from build123d import *

# Parameters (mm, degrees)
SKETCH2_W                  = 254
SKETCH2_H                  = 88.9
RECTANGLE_EXTRUSION_DEPTH  = 12.7
SKETCH4_W                  = 12.7
SKETCH4_H                  = 12.7
FRONT_FACE_TABS_DEPTH      = 12.7
SKETCH6_R                  = 2.24536
TAB_CURVE_FRONT_BACK_DEPTH = 12.7
SKETCH7_W                  = 12.7
SKETCH7_H                  = 12.7
RIGHT_FACE_TABS_DEPTH      = 12.7
SKETCH8_R                  = 2.24536
TAB_CURVE_LEFT_RIGHT_DEPTH = 12.7
SKETCH9_R                  = 2.5527
NUT_STRIPS_CUT_DEPTH       = 152.471127612


with BuildPart() as part:
    # Sketch2 → Rectangle Extrusion (new body)
    with BuildSketch(Plane(origin=(0, 0, 0), x_dir=(1, 0, 0), z_dir=(0, 1, 0))):
        Rectangle(SKETCH2_W, SKETCH2_H)
    extrude(amount=RECTANGLE_EXTRUSION_DEPTH)

    # Sketch4 → Front Face Tabs (add)
    with BuildSketch(Plane.XY.offset(44.45)):
        with Locations((-63.5, 6.35)):
            Rectangle(SKETCH4_W, SKETCH4_H)
        with Locations((63.5, 6.35)):
            Rectangle(SKETCH4_W, SKETCH4_H)
    front_face_tabs = extrude(amount=FRONT_FACE_TABS_DEPTH)

    # Mirror Rear Face Tabs: Front Face Tabs across plane
    add(front_face_tabs.mirror(Plane.XY))

    # Sketch6 → Tab Curve Front Back (cut)
    with BuildSketch(Plane(origin=(0, 12.7, 0), x_dir=(1, 0, 0), z_dir=(0, 1, 0))):
        with Locations((-71.4375, 46.0375)):
            Circle(SKETCH6_R)
        with Locations((-55.5625, 46.0375)):
            Circle(SKETCH6_R)
        with Locations((55.5625, 46.0375)):
            Circle(SKETCH6_R)
        with Locations((71.4375, 46.0375)):
            Circle(SKETCH6_R)
        with Locations((71.4375, -46.0375)):
            Circle(SKETCH6_R)
        with Locations((55.5625, -46.0375)):
            Circle(SKETCH6_R)
        with Locations((-55.5625, -46.0375)):
            Circle(SKETCH6_R)
        with Locations((-71.4375, -46.0375)):
            Circle(SKETCH6_R)
    extrude(amount=-TAB_CURVE_FRONT_BACK_DEPTH, mode=Mode.SUBTRACT)

    # Sketch7 → Right Face Tabs (add)
    with BuildSketch(Plane(origin=(127, 0, 0), x_dir=(0, 0, -1), z_dir=(1, 0, 0))):
        with Locations((-19.05, 6.35)):
            Rectangle(SKETCH7_W, SKETCH7_H)
        with Locations((19.05, 6.35)):
            Rectangle(SKETCH7_W, SKETCH7_H)
    right_face_tabs = extrude(amount=RIGHT_FACE_TABS_DEPTH)

    # Mirror Left Face Tabs: Right Face Tabs across plane
    add(right_face_tabs.mirror(Plane(origin=(0, 0, 0), x_dir=(0, 0, 1), z_dir=(1, 0, 0))))

    # Sketch8 → Tab Curve Left Right (cut)
    with BuildSketch(Plane(origin=(0, 12.7, 0), x_dir=(1, 0, 0), z_dir=(0, 1, 0))):
        with Locations((128.5875, 26.9875)):
            Circle(SKETCH8_R)
        with Locations((128.5875, 11.1125)):
            Circle(SKETCH8_R)
        with Locations((128.5875, -11.1125)):
            Circle(SKETCH8_R)
        with Locations((128.5875, -26.9875)):
            Circle(SKETCH8_R)
        with Locations((-128.5875, -26.9875)):
            Circle(SKETCH8_R)
        with Locations((-128.5875, -11.1125)):
            Circle(SKETCH8_R)
        with Locations((-128.5875, 11.1125)):
            Circle(SKETCH8_R)
        with Locations((-128.5875, 26.9875)):
            Circle(SKETCH8_R)
    extrude(amount=-TAB_CURVE_LEFT_RIGHT_DEPTH, mode=Mode.SUBTRACT)

    # Sketch9 → Nut Strips Cut (cut, through all)
    with BuildSketch(Plane.XZ):
        with Locations(Location((-107.95, 38.1, 0), (0, 0, 270))):
            Circle(SKETCH9_R)
        with Locations(Location((-120.65, 25.4, 0), (0, 0, 270))):
            Circle(SKETCH9_R)
        with Locations(Location((-120.65, 6.35, 0), (0, 0, 270))):
            Circle(SKETCH9_R)
        with Locations(Location((-120.65, -12.7, 0), (0, 0, 270))):
            Circle(SKETCH9_R)
        with Locations(Location((-120.65, -31.75, 0), (0, 0, 270))):
            Circle(SKETCH9_R)
        with Locations(Location((-88.9, 38.1, 0), (0, 0, 270))):
            Circle(SKETCH9_R)
        with Locations(Location((-69.85, 38.1, 0), (0, 0, 270))):
            Circle(SKETCH9_R)
        with Locations(Location((-50.8, 38.1, 0), (0, 0, 270))):
            Circle(SKETCH9_R)
        with Locations(Location((-31.75, 38.1, 0), (0, 0, 270))):
            Circle(SKETCH9_R)
        with Locations(Location((-12.7, 38.1, 0), (0, 0, 270))):
            Circle(SKETCH9_R)
        with Locations(Location((6.35, 38.1, 0), (0, 0, 270))):
            Circle(SKETCH9_R)
        with Locations(Location((25.4, 38.1, 0), (0, 0, 270))):
            Circle(SKETCH9_R)
        with Locations(Location((44.45, 38.1, 0), (0, 0, 270))):
            Circle(SKETCH9_R)
        with Locations(Location((63.5, 38.1, 0), (0, 0, 270))):
            Circle(SKETCH9_R)
        with Locations(Location((82.55, 38.1, 0), (0, 0, 270))):
            Circle(SKETCH9_R)
        with Locations(Location((101.6, 38.1, 0), (0, 0, 270))):
            Circle(SKETCH9_R)
        with Locations(Location((107.95, -38.1, 0), (0, 0, 270))):
            Circle(SKETCH9_R)
        with Locations(Location((120.65, -25.4, 0), (0, 0, 270))):
            Circle(SKETCH9_R)
        with Locations(Location((120.65, -6.35, 0), (0, 0, 270))):
            Circle(SKETCH9_R)
        with Locations(Location((120.65, 12.7, 0), (0, 0, 270))):
            Circle(SKETCH9_R)
        with Locations(Location((120.65, 31.75, 0), (0, 0, 270))):
            Circle(SKETCH9_R)
        with Locations(Location((88.9, -38.1, 0), (0, 0, 270))):
            Circle(SKETCH9_R)
        with Locations(Location((69.85, -38.1, 0), (0, 0, 270))):
            Circle(SKETCH9_R)
        with Locations(Location((50.8, -38.1, 0), (0, 0, 270))):
            Circle(SKETCH9_R)
        with Locations(Location((31.75, -38.1, 0), (0, 0, 270))):
            Circle(SKETCH9_R)
        with Locations(Location((12.7, -38.1, 0), (0, 0, 270))):
            Circle(SKETCH9_R)
        with Locations(Location((-6.35, -38.1, 0), (0, 0, 270))):
            Circle(SKETCH9_R)
        with Locations(Location((-25.4, -38.1, 0), (0, 0, 270))):
            Circle(SKETCH9_R)
        with Locations(Location((-44.45, -38.1, 0), (0, 0, 270))):
            Circle(SKETCH9_R)
        with Locations(Location((-63.5, -38.1, 0), (0, 0, 270))):
            Circle(SKETCH9_R)
        with Locations(Location((-82.55, -38.1, 0), (0, 0, 270))):
            Circle(SKETCH9_R)
        with Locations(Location((-101.6, -38.1, 0), (0, 0, 270))):
            Circle(SKETCH9_R)
    extrude(amount=-NUT_STRIPS_CUT_DEPTH, mode=Mode.SUBTRACT)


solid = part.part
The listing builds one solid part. Answer for the finished solid, in the listing's coordinates (mm). A direction names the side the tool comes from. Give positions to 0.01 mm unless a question says otherwise; leave off trailing zeros. Order: outer loops, then holes, each group sorted by start corner. A loop starts at its lowest first (then second) coordinate and runs counter-clockwise, first axis right, second up. Notation, with made-up numbers: (-27, 26.5) - (-1, 26.5) arc R36 ccw to (-1, 62.5) - close; hole circle Ø1 at (48.25, 62.25). An arc over 180 degrees is marked (long way). One line per item, written item: value. Start each with the question number.
1) The mould has two halves that part along Z. Classify faces 1 (the face through (-64, 6, 57.15)), 2 (the face through (-110.442, 6.261, 38.653)), 3 (the face through (-57.15, 6, -52)): released by +Z, released by -Z, zero draft, split by the parting line, or undercut.
2) Given pin 1 Ø3 at (x, y) = (134.5, 7.5) entering from +Z; pin 2 Ø3 at (y, z) = (5, -54.5) entering from -X; pin 3 Ø3 at (x, y) = (9.5, 4.5) entering from -Z, each flat-ended and moving along its own axis, determine where each tip first touches the part or whether it passes through.
3) Find the intervals of material crossed by L1, parallel to X at y = 4.75, z = 31.75; L2, parallel to X at y = 9.75, z = 25; L3, parallel to Z at x = 123, y = 6, in increasing order.
4) A cutting plane is placed at C-C on x = 63.5. Give the vertices of the cut face in (y, z), then the cut area to 3 significant figures.
5) A cutting plane is placed at B-B on z = 6.35. Give the vertices of the cut face in (x, y).
6) A tool of negligible diameter and unlimited length cuts with its end or side. For faces 4 (the face through (127, 6, 0)), 5 (the face through (-57.15, 6, 52)), 6 (the face through (-135, 6, 12.7)), 7 (the face through (-1, 6, -44.45)), 8 (the face through (-127, 6, 37)), from which of +Z, -Z, +X, -X, +Y, -Y can it reach the whole face along a straight path? Write none if from no direction.
7) A cutting plane is placed at D-D on y = 8.5. State how many separate pieces and enclosed holes the cut face has, then the cut area to 3 significant figures.
8) A cutting plane is placed at A-A on x = -120.65. Give the vertices of the cut face in (y, z), then the cut area to 3 significant figures.
Answer sheet:
1. face 1: released by +Z
1. face 2: undercut
1. face 3: zero draft
2. pin 1: stops at z = 25.4
2. pin 2: stops at x = -69.85
2. pin 3: stops at z = -44.45
3. L1: x = -127 to 118.1, 123.2 to 127
3. L2: x = -139.7 to -129.63, -127.54 to -123.17, -118.13 to 127.54, 129.63 to 139.7
3. L3: z = -44.45 to -26.4, -24.4 to -7.35, -5.35 to 11.7, 13.7 to 30.75, 32.75 to 44.45
4. outline: (0, -57.15) - (12.7, -57.15) - (12.7, 35.55) - (0, 35.55) - close; (0, 40.65) - (12.7, 40.65) - (12.7, 57.15) - (0, 57.15) - close
4. area: 1,390 mm2
5. outline: (-127, 0) - (-123.2, 0) - (-123.2, 12.7) - (-127, 12.7) - close; (-118.1, 0) - (127, 0) - (127, 12.7) - (-118.1, 12.7) - close
6. face 4: +X, +Y, -Y
6. face 5: +Z, +Y, -Y
6. face 6: -X, +Y, -Y
6. face 7: -Z, +Y, -Y
6. face 8: +Z, -X, +Y, -Y
7. separate pieces: 1
7. enclosed holes: 32
7. area: 23,200 mm2
8. outline: (0, -44.45) - (12.7, -44.45) - (12.7, -34.3) - (0, -34.3) - close; (0, -29.2) - (12.7, -29.2) - (12.7, -15.25) - (0, -15.25) - close; (0, -10.15) - (12.7, -10.15) - (12.7, 3.8) - (0, 3.8) - close; (0, 8.9) - (12.7, 8.9) - (12.7, 22.85) - (0, 22.85) - close; (0, 27.95) - (12.7, 27.95) - (12.7, 44.45) - (0, 44.45) - close
8. area: 870 mm2
